```python
from build123d import *

# Parameters (mm, degrees)
BOSS_EXTRUDE1_DEPTH = 25
SKETCH2_OUTSIDE_W   = 142.428
SKETCH2_OUTSIDE_H   = 151.71
SKETCH2_OUTSIDE_R   = 29.999119987
CUT_EXTRUDE2_DEPTH  = 53.200352489
CUT_EXTRUDE2_DRAFT  = -30


with BuildPart() as part:
    # Sketch1 → Boss-Extrude1 (new body)
    with BuildSketch(Plane.XY):
        Polygon((0, -34.64), (29.999119987, -17.32), (29.999119987, 17.32), (0, 34.64), (-29.999119987, 17.32), (-29.999119987, -17.32), align=None)
    extrude(amount=BOSS_EXTRUDE1_DEPTH)


with BuildPart() as cut_extrude2_tool:
    # Sketch2 outside → Cut-Extrude2 (with draft: the straight prism first)
    with BuildSketch(Plane.XY.offset(25)):
        Rectangle(SKETCH2_OUTSIDE_W, SKETCH2_OUTSIDE_H)
        Circle(SKETCH2_OUTSIDE_R, mode=Mode.SUBTRACT)
    extrude(amount=-CUT_EXTRUDE2_DEPTH)
    # Cut-Extrude2: the draft: its side faces are tilted about the plane it starts from
    cut_extrude2_sides = [cut_extrude2_tool.faces().sort_by_distance(p)[0] for p in [
        (0, -75.855, -1.600176245),
        (71.214, 0, -1.600176245),
        (0, 75.855, -1.600176245),
        (-71.214, 0, -1.600176245),
        (-29.999119987, 0, -1.600176245),
    ]]
    draft(cut_extrude2_sides, Plane.XY.offset(25), CUT_EXTRUDE2_DRAFT)


with BuildPart() as part_1:
    add(part.part)

    # Cut-Extrude2: cut by cut_extrude2_tool
    add(cut_extrude2_tool.part, mode=Mode.SUBTRACT)


solid = part_1.part
```
Check sheet for the modelled part. Datum: model origin and axes. Units: mm. Round coordinates to 2 decimals unless told otherwise and drop trailing zeros. Loops run counter-clockwise (first coordinate to the right, second up) from the corner with the lowest first, then second, coordinate; pieces in that order, holes last. Notation, with made-up numbers: (-21.75, 27) - (36.25, 27) arc R23 ccw to (36.25, 60) - close; hole circle Ø5 at (57, -3). An arc over 180 degrees is marked (long way). Answer as a JSON object with one key per item and string values. Group by question number.
Q1. Sectioned sample at B-B, the plane z = 14.5. Enter the section's corners in (x, y), plus the area to 3 significant figures.
Q2. Scan lines: line 1 along X through (y, z) = (20.5, 1); line 2 along Y through (x, z) = (-4, 3.5); line 3 along Y through (x, z) = (-10, 15.25). Record each from-to range of solid material in increasing order. Write a range as [from, to].
Q3. Gauge pin test, flat ends, axial feed: P1, Ø5, axis at y = -19, z = 2.5, coming from the +X side; P2, Ø12, axis at x = -23, z = 8, coming from the -Y side; P3, Ø5, axis at x = -6.5, z = 17, coming from the -Y side; P4, Ø6, axis at y = -21, z = 21.5, coming from the +X side. Record the tip position at first contact, or that the pin passes through.
Q4. Sectioned sample at A-A, the plane z = 20. Enter the section's corners in (x, y), plus the area to 3 significant figures.
Solution:
{
 "1": {"outline": "(-30, -17.32) - (0, -34.64) - (30, -17.32) - (30, 17.32) - (0, 34.64) - (-30, 17.32) - close", "area": "3,120 mm²"},
 "2": {"line 1": "x = [-24.49, 24.49]", "line 2": "y = [-32.33, 32.33]", "line 3": "y = [-28.87, 28.87]"},
 "3": {"P1": "stops at x = 30", "P2": "stops at y = -24.83", "P3": "stops at y = -32.33", "P4": "stops at x = 27.36"},
 "4": {"outline": "(-30, -13.47) arc R32.89 ccw to (-26.67, -19.24) - (-3.33, -32.72) arc R32.89 ccw to (3.33, -32.72) - (26.67, -19.24) arc R32.89 ccw to (30, -13.47) - (30, 13.47) arc R32.89 ccw to (26.67, 19.24) - (3.33, 32.72) arc R32.89 ccw to (-3.33, 32.72) - (-26.67, 19.24) arc R32.89 ccw to (-30, 13.47) - close", "area": "3,080 mm²"}
}
